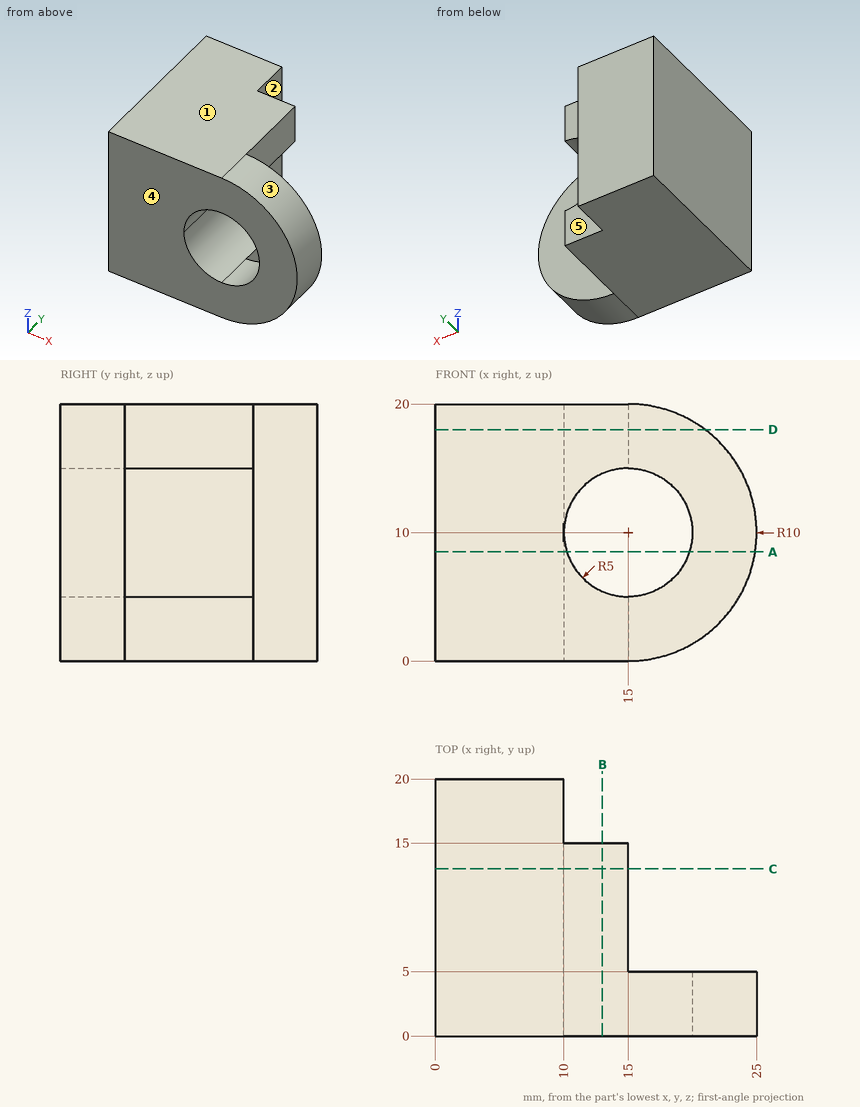
Geometry check sheet. Reference: drawing and pictorial views, mm from the part's lowest x, y, z. A direction names the side the tool comes from. Round coordinates to 2 decimals unless told otherwise and drop trailing zeros. Write each loop counter-clockwise with the first axis right and the second up, starting at its lowest first coordinate (ties: lowest second). Pieces come first, ordered by that corner, then holes. Notation, with made-up numbers: (18.5, 34) -> (59.5, 34) arc R28 ccw to (59.5, 65) -> close; hole circle Ø10 at (3.5, 34). An arc over 180 degrees is marked (long way). Answer as CSV lines item,"result". Start each with the question number.
1) Tool access check on the marked faces 1 and 2. Record the directions out of +Z, -Z, +X, -X, +Y, -Y that give a thin tool (end or side, any length) a straight path to the whole face; none if there is none.
2) Section check C-C on y = 13. Enter the section's corners in (x, z).
3) Go/stop test with flat-tipped pins: P1, Ø2, axis at y = 12, z = 4.5, coming from the -X side; P2, Ø3, axis at x = 20.5, y = 4, coming from the +Z side; P3, Ø4, axis at y = 10.5, z = 17.5, coming from the +X side; P4, Ø8, axis at x = 22.5, z = 12, coming from the +Y side. Record where each tip stops, or that it passes through.
4) Release check for a two-part mould opening along Y. For the marked faces 3, 4 and 5 record: pulls with the +Y half, pulls with the -Y half, needs draft (parallel to the pull), parting line crosses it, or undercut.
5) Section check A-A on z = 8.5. Enter the section's corners in (x, y).
6) Material ranges on line 1 (Y direction, x = 20.5, z = 9); line 2 (Z direction, x = 12.5, y = 2); line 3 (Z direction, x = 15.5, y = 1), recorded low to high. Write a range as from..to.
7) Section check D-D on z = 18. Enter the section's corners in (x, y), and give its area (3 significant figures).
8) Section check B-B on x = 13. Enter the section's corners in (y, z).
Found:
1,face 1,"+Z, +X, -X, +Y, -Y"
1,face 2,"+Z, -Z, +X, +Y"
2,outline,"(0, 0) -> (15, 0) -> (15, 5) arc R5 cw to (15, 15) -> (15, 20) -> (0, 20) -> close"
3,P1,"stops at x = 0"
3,P2,"stops at z = 19.17"
3,P3,"stops at x = 15"
3,P4,"stops at y = 5"
4,face 3,"needs draft"
4,face 4,"pulls with the -Y half"
4,face 5,"pulls with the +Y half"
5,outline,"(0, 0) -> (10.23, 0) -> (10.23, 15) -> (10, 15) -> (10, 20) -> (0, 20) -> close; (19.77, 0) -> (24.89, 0) -> (24.89, 5) -> (19.77, 5) -> close"
6,line 1,"y = 0..5"
6,line 2,"z = 0..5.67, 14.33..20"
6,line 3,"z = 0.01..5.03, 14.97..19.99"
7,outline,"(0, 0) -> (21, 0) -> (21, 5) -> (15, 5) -> (15, 15) -> (10, 15) -> (10, 20) -> (0, 20) -> close"
7,area,"305 mm^2"
8,outline,"(0, 0) -> (15, 0) -> (15, 5.42) -> (0, 5.42) -> close; (0, 14.58) -> (15, 14.58) -> (15, 20) -> (0, 20) -> close"
